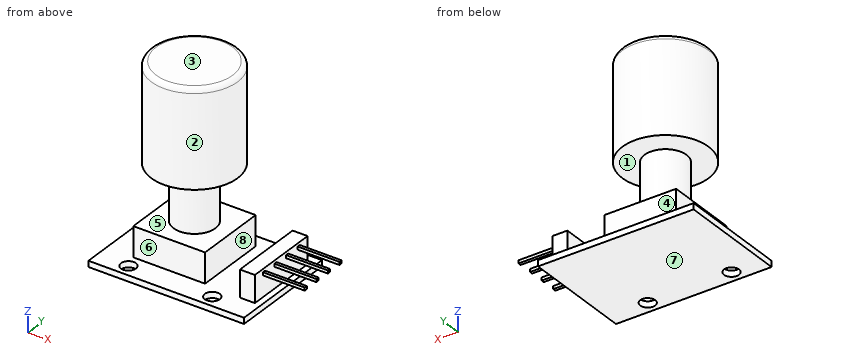
```python
from build123d import *

# Parameters (mm, degrees)
F0_W      = 26
F0_H      = 18.5
F0_R      = 1.25
F1_DEPTH  = 1
F2_W      = 12
F2_H      = 12
F3_DEPTH  = 5
F4_R      = 3.5
F5_DEPTH  = 9.3
F6_R      = 7.2
F7_DEPTH  = 16.2
F8_R      = 0.8
F9_W      = 2.5
F9_H      = 12.5
F10_DEPTH = 4.5
F11_W     = 0.5
F11_H     = 0.5
F12_DEPTH = 7


with BuildPart() as f1:
    # F0 (on Top) → F1 (new body)
    with BuildSketch(Plane.XY):
        Rectangle(F0_W, F0_H)
        with Locations((-7.75, -7.2)):
            Circle(F0_R, mode=Mode.SUBTRACT)
        with Locations((6.25, -7.2)):
            Circle(F0_R, mode=Mode.SUBTRACT)
    extrude(amount=F1_DEPTH)

    # F2 (on face) → F3 (join)
    with BuildSketch(Plane.XY.offset(1)):
        with Locations((-2.5, 1)):
            Rectangle(F2_W, F2_H)
    extrude(amount=F3_DEPTH)

    # F4 (on face) → F5 (join)
    with BuildSketch(Plane.XY.offset(6)):
        with Locations((-2.5, 1)):
            Circle(F4_R)
    extrude(amount=F5_DEPTH)

    # F6 (on face) → F7 (join)
    with BuildSketch(Plane.XY.offset(15.3)):
        with Locations((-2.5, 1)):
            Circle(F6_R)
    extrude(amount=F7_DEPTH)

    # F8
    f8_edges = [f1.edges().sort_by_distance(p)[0] for p in [
        (-9.7, 1, 31.5),
    ]]
    fillet(f8_edges, radius=F8_R)

    # F9 (on face) → F10 (join)
    with BuildSketch(Plane.XY.offset(1)):
        with Locations((10.75, 1)):
            Rectangle(F9_W, F9_H)
    extrude(amount=F10_DEPTH)

    # F11 (on face) → F12 (join)
    with BuildSketch(Plane.YZ.offset(12)):
        with Locations((-3.125, 4.757234)):
            Rectangle(F11_W, F11_H)
        with Locations((-0.375, 4.757234)):
            Rectangle(F11_W, F11_H)
        with Locations((2.375, 4.757234)):
            Rectangle(F11_W, F11_H)
        with Locations((5.125, 4.757234)):
            Rectangle(F11_W, F11_H)
    extrude(amount=F12_DEPTH)


solid = f1.part
```
Geometry: final body of the model. Coordinates: model frame, mm. Face numbers are marked on the shaded views. A direction names the side the tool comes from. Round coordinates to 2 decimals unless told otherwise and drop trailing zeros. Order: outer loops, then holes, each group sorted by start corner. A loop starts at its lowest first (then second) coordinate and runs counter-clockwise, first axis right, second up. Notation, with made-up numbers: (56.5, 37.25) - (106.5, 37.25) arc R16 cw to (106.5, 48.25) - close; hole circle Ø5 at (-21, 17). An arc over 180 degrees is marked (long way). Use CSV: the item, a comma, the result in double quotes. Start each with the question number.
Q1. Section query D-D (y = 1). Return loops of the section in (x, z).
Q2. Material intervals for line 1 along Z through (x, y) = (3, 1.5); line 2 along X through (y, z) = (-1.25, 3.5); line 3 along Y through (x, z) = (6.25, 0.6), sorted ascending. Write a range as from..to.
Q3. Access query for the marked faces 5, 6, 7 and 8. Directions: +Z, -Z, +X, -X, +Y, -Y. A direction counts if a zero-diameter tool reaches every point of the face in a straight line with its end or side. Return the directions, or none.
Q4. Section query A-A (z = 2). Return loops of the section in (x, y).
Q5. Section query C-C (x = 6.25). Return loops of the section in (y, z).
Q6. Mould query, pull axis Z, two halves, no side actions, for the marked faces 1, 2, 3 and 4. Classes: +Z half, -Z half, draft (parallel to the pull), parting line (faces both ways), or undercut.
Q7. Section query B-B (y = -7.2). Return loops of the section in (x, z), and give its area (3 significant figures).
Q8. First-contact query: pin 1 (1.5 mm diameter, centred on x = -3.5, z = 4, fed in from +Y); pin 2 (1.2 mm diameter, centred on x = 10.5, z = 4, fed in from -Y); pin 3 (2 mm diameter, centred on x = -2, z = 17, fed in from -Y). Flat tips, straight axial feed; report the tip coordinate or a pass-through.
Result set:
1,outline,"(-13, 0) - (13, 0) - (13, 1) - (12, 1) - (12, 5.5) - (9.5, 5.5) - (9.5, 1) - (3.5, 1) - (3.5, 6) - (1, 6) - (1, 15.3) - (4.7, 15.3) - (4.7, 30.7) arc R0.8 ccw to (3.9, 31.5) - (-8.9, 31.5) arc R0.8 ccw to (-9.7, 30.7) - (-9.7, 15.3) - (-6, 15.3) - (-6, 6) - (-8.5, 6) - (-8.5, 1) - (-13, 1) - close"
2,line 1,"z = 0..6, 15.3..31.5"
2,line 2,"x = -8.5..3.5, 9.5..12"
2,line 3,"y = -9.25..-8.45, -5.95..9.25"
3,face 5,"none"
3,face 6,"-X, -Y"
3,face 7,"-Z, +X, -X, +Y, -Y"
3,face 8,"+Y, -Y"
4,outline,"(-8.5, -5) - (3.5, -5) - (3.5, 7) - (-8.5, 7) - close; (9.5, -5.25) - (12, -5.25) - (12, 7.25) - (9.5, 7.25) - close"
5,outline,"(-9.25, 0) - (-8.45, 0) - (-8.45, 1) - (-9.25, 1) - close; (-5.95, 0) - (9.25, 0) - (9.25, 1) - (-5.95, 1) - close"
6,face 1,"undercut"
6,face 2,"draft"
6,face 3,"+Z half"
6,face 4,"undercut"
7,outline,"(-13, 0) - (-9, 0) - (-9, 1) - (-13, 1) - close; (-6.5, 0) - (5, 0) - (5, 1) - (-6.5, 1) - close; (7.5, 0) - (13, 0) - (13, 1) - (7.5, 1) - close"
7,area,"21.0 mm2"
8,pin 1,"stops at y = 7"
8,pin 2,"stops at y = -5.25"
8,pin 3,"stops at y = -6.2"
